Build history of the part. All positions in model axes, mm. Give positions to 0.01 mm unless a question says otherwise; leave off trailing zeros. Loops run counter-clockwise (first coordinate to the right, second up) from the corner with the lowest first, then second, coordinate; pieces in that order, holes last. Notation, with made-up numbers: (31, 72.25) - (82, 72.25) arc R10 ccw to (82, 80.25) - close; hole circle Ø3 at (-18, 25.5). An arc over 180 degrees is marked (long way). Return JSON: item names as keys, results as strings. Group by question number.
1) Slice it at C-C (z = 25). List the corners of the cut face in (x, y), and give its area (3 significant figures).
2) Slice it at A-A (x = 0). List the corners of the cut face in (y, z), and give its area (3 significant figures).
3) Drill centre lines: probe 1 along X at (y, z) = (0.25, 14); probe 2 along X at (y, z) = (1.25, 32); probe 3 along Y at (x, z) = (-0.5, 28.5). Where is each one in solid material? Low to high. Write a range as from..to.
4) Slice it at D-D (z = 4.5). List the corners of the cut face in (x, y).
5) Slice it at B-B (y = 0). List the corners of the cut face in (x, z), and give its area (3 significant figures).
```python
from build123d import *

# Parameters (mm, degrees)
F0_R       = 4
F1_DEPTH   = 35
F2_SIZE2   = 7
F2_SIZE    = 0.5
F2_2_SIZE2 = 7
F2_2_SIZE  = 0.5
F3_W       = 10
F3_H       = 35
F4_DEPTH   = 12.5


with BuildPart() as f1:
    # F0 (on Top) → F1 (new body)
    with BuildSketch(Plane.XY):
        Circle(F0_R)
    extrude(amount=F1_DEPTH)

    # F2
    f2_edges = [f1.edges().sort_by_distance(p)[0] for p in [
        (-4, 0, 35),
    ]]
    f2_side = f1.faces().sort_by_distance((0, 0, 35))[0]
    chamfer(f2_edges, length=F2_SIZE, length2=F2_SIZE2, reference=f2_side)

    # F2#2
    f2_2_edges = [f1.edges().sort_by_distance(p)[0] for p in [
        (-4, 0, 0),
    ]]
    f2_2_side = f1.faces().sort_by_distance((0, 0, 0))[0]
    chamfer(f2_2_edges, length=F2_2_SIZE, length2=F2_2_SIZE2, reference=f2_2_side)

    # F3 (on Right) → F4 (cut, symmetric)
    with BuildSketch(Plane.YZ):
        with Locations((8.9, 17.5)):
            Rectangle(F3_W, F3_H)
    extrude(amount=F4_DEPTH, both=True, mode=Mode.SUBTRACT)


solid = f1.part
```
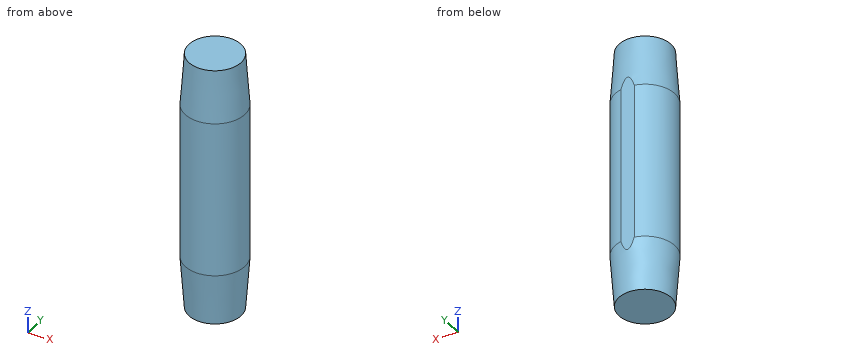
Results:
{
 "1": {"outline": "(-0.89, 3.9) arc R4 ccw (long way) to (0.89, 3.9) - close", "area": "50.1 mm2"},
 "2": {"outline": "(-4, 7) - (-3.5, 0) - (3.5, 0) - (3.9, 5.6) - (3.9, 29.4) - (3.5, 35) - (-3.5, 35) - (-4, 28) - close", "area": "271 mm2"},
 "3": {"probe 1": "-3.99..3.99", "probe 2": "-3.5..3.5", "probe 3": "-3.93..3.9"},
 "4": {"outline": "circle Ø7.64 at (0, 0)"},
 "5": {"outline": "(-4, 7) - (-3.5, 0) - (3.5, 0) - (4, 7) - (4, 28) - (3.5, 35) - (-3.5, 35) - (-4, 28) - close", "area": "273 mm2"}
}
